For this review, take the finished solid that the model builds, in its own axes (mm). A direction names the side the tool comes from. Round coordinates to 2 decimals unless told otherwise and drop trailing zeros. Order: outer loops, then holes, each group sorted by start corner. A loop starts at its lowest first (then second) coordinate and runs counter-clockwise, first axis right, second up.
```python
from build123d import *

# Parameters (mm, degrees)
EXTRUDE_1_DEPTH     = 1.5
EXTRUDE_2_DEPTH     = 6.5
CUT_EXTRUDE_1_DEPTH = 1
SKETCH_4_R          = 4.015
EXTRUDE_3_DEPTH     = 4
SKETCH_6_R          = 4.015
EXTRUDE_4_DEPTH     = 4
SKETCH_7_R          = 2.4
CUT_EXTRUDE_3_DEPTH = 48.711742668
SKETCH_8_W          = 9
SKETCH_8_H          = 5
EXTRUDE_5_DEPTH     = 8.5
SKETCH_9_W          = 4.5
SKETCH_9_H          = 5
SKETCH_10_R         = 1.75
CUT_EXTRUDE_4_DEPTH = 51.943190951


with BuildPart() as part:
    # 스케치1 → 보스-돌출1 (new body)
    with BuildSketch(Plane(origin=(0, 0, 0), x_dir=(1, 0, 0), z_dir=(0, 1, 0))):
        Polygon((13.776603565, 33.25966317), (-13.776603565, 33.25966317), (-33.25966317, 13.776603565), (-33.25966317, -13.776603565), (-13.776603565, -33.25966317), (13.776603565, -33.25966317), (33.25966317, -13.776603565), (33.25966317, 13.776603565), align=None)
        Polygon((-13.27954729, 32.05966317), (-32.05966317, 13.27954729), (-32.05966317, -13.27954729), (-13.27954729, -32.05966317), (13.27954729, -32.05966317), (32.05966317, -13.27954729), (32.05966317, 13.27954729), (13.27954729, 32.05966317), align=None, mode=Mode.SUBTRACT)
        Polygon((13.27954729, 32.05966317), (-13.27954729, 32.05966317), (-32.05966317, 13.27954729), (-32.05966317, -13.27954729), (-13.27954729, -32.05966317), (13.27954729, -32.05966317), (32.05966317, -13.27954729), (32.05966317, 13.27954729), align=None)
    extrude(amount=EXTRUDE_1_DEPTH)

    # 스케치2 → 보스-돌출2 (add)
    with BuildSketch(Plane.XZ):
        Polygon((-33.25966317, -13.776603565), (-13.776603565, -33.25966317), (13.776603565, -33.25966317), (33.25966317, -13.776603565), (33.25966317, 13.776603565), (13.776603565, 33.25966317), (-13.776603565, 33.25966317), (-33.25966317, 13.776603565), align=None)
        Polygon((-32.05966317, -13.27954729), (-13.27954729, -32.05966317), (13.27954729, -32.05966317), (32.05966317, -13.27954729), (32.05966317, 13.27954729), (13.27954729, 32.05966317), (-13.27954729, 32.05966317), (-32.05966317, 13.27954729), align=None, mode=Mode.SUBTRACT)
        Polygon((-32.05966317, 13.27954729), (-32.05966317, -13.27954729), (-13.27954729, -32.05966317), (13.27954729, -32.05966317), (32.05966317, -13.27954729), (32.05966317, 13.27954729), (13.27954729, 32.05966317), (-13.27954729, 32.05966317), align=None)
        Polygon((-30.85966317, -12.782491015), (-12.782491015, -30.85966317), (12.782491015, -30.85966317), (30.85966317, -12.782491015), (30.85966317, 12.782491015), (12.782491015, 30.85966317), (-12.782491015, 30.85966317), (-30.85966317, 12.782491015), align=None, mode=Mode.SUBTRACT)
        Polygon((-30.85966317, 12.782491015), (-30.85966317, -12.782491015), (-12.782491015, -30.85966317), (12.782491015, -30.85966317), (30.85966317, -12.782491015), (30.85966317, 12.782491015), (12.782491015, 30.85966317), (-12.782491015, 30.85966317), align=None)
        Polygon((-29.65966317, -12.285434741), (-12.285434741, -29.65966317), (12.285434741, -29.65966317), (29.65966317, -12.285434741), (29.65966317, 12.285434741), (12.285434741, 29.65966317), (-12.285434741, 29.65966317), (-29.65966317, 12.285434741), align=None, mode=Mode.SUBTRACT)
    extrude(amount=EXTRUDE_2_DEPTH)

    # 스케치3 → 컷-돌출1 (cut)
    with BuildSketch(Plane.XZ.offset(6.5)):
        Polygon((-32.05966317, -13.27954729), (-13.27954729, -32.05966317), (13.27954729, -32.05966317), (32.05966317, -13.27954729), (32.05966317, 13.27954729), (13.27954729, 32.05966317), (-13.27954729, 32.05966317), (-32.05966317, 13.27954729), align=None)
        Polygon((-30.85966317, -12.782491015), (-12.782491015, -30.85966317), (12.782491015, -30.85966317), (30.85966317, -12.782491015), (30.85966317, 12.782491015), (12.782491015, 30.85966317), (-12.782491015, 30.85966317), (-30.85966317, 12.782491015), align=None, mode=Mode.SUBTRACT)
    extrude(amount=-CUT_EXTRUDE_1_DEPTH, mode=Mode.SUBTRACT)

    # 스케치4 → 보스-돌출3 (add)
    with BuildSketch(Plane(origin=(0, 1.5, 0), x_dir=(1, 0, 0), z_dir=(0, 1, 0))):
        with Locations(Location((0, 0, 0), (0, 0, 270))):
            Circle(SKETCH_4_R)
    extrude(amount=EXTRUDE_3_DEPTH)

    # 스케치6 → 보스-돌출4 (add)
    with BuildSketch(Plane.XZ):
        with Locations(Location((0, 0, 0), (0, 0, 90))):
            Circle(SKETCH_6_R)
    extrude(amount=EXTRUDE_4_DEPTH)

    # 스케치7 → 컷-돌출3 (cut, through all)
    with BuildSketch(Plane(origin=(0, 1.5, 0), x_dir=(1, 0, 0), z_dir=(0, 1, 0))):
        with Locations(Location((0, -27, 0), (0, 0, 270))):
            Circle(SKETCH_7_R)
    extrude(amount=-CUT_EXTRUDE_3_DEPTH, mode=Mode.SUBTRACT)

    # 스케치8 → 보스-돌출5 (add)
    with BuildSketch(Plane(origin=(0, 1.5, 0), x_dir=(1, 0, 0), z_dir=(0, 1, 0))):
        with Locations((-28.75966317, 0)):
            Rectangle(SKETCH_8_W, SKETCH_8_H)
    extrude_5 = extrude(amount=EXTRUDE_5_DEPTH)

    # 스케치9 → 회전1 (revolve)
    with BuildSketch(Plane(origin=(0, 10, 0), x_dir=(1, 0, 0), z_dir=(0, 1, 0))):
        with Locations((-31.00966317, 0)):
            Rectangle(SKETCH_9_W, SKETCH_9_H)
    revolve_1 = revolve(axis=Axis((-28.75966317, 10, -5.508751215), (0, 0, 1)))

    # 스케치10 → 컷-돌출4 (cut, through all)
    with BuildSketch(Plane.XY.offset(2.5)):
        with Locations((-28.75966317, 10)):
            Circle(SKETCH_10_R)
    cut_extrude_4 = extrude(amount=-CUT_EXTRUDE_4_DEPTH, mode=Mode.SUBTRACT)

    # 대칭 복사1: 보스-돌출5, 회전1, 컷-돌출4 across plane
    add(extrude_5.mirror(Plane(origin=(0, 0, 0), x_dir=(0, 0, 1), z_dir=(1, 0, 0))))
    add(revolve_1.mirror(Plane(origin=(0, 0, 0), x_dir=(0, 0, 1), z_dir=(1, 0, 0))))
    add(cut_extrude_4.mirror(Plane(origin=(0, 0, 0), x_dir=(0, 0, 1), z_dir=(1, 0, 0))), mode=Mode.SUBTRACT)


solid = part.part
```
Q1. Take a section at D-D, the plane z = 27. State the section outline as (x, y) points, plus the area to 3 significant figures.
Q2. Take a section at B-B, the plane z = 0. Count the separate pieces of the cut face and the enclosed holes in it, plus the area to 3 significant figures.
Q3. Clearance check with flat-ended pins moving along their axes: pin 1 (4.5 mm diameter, centred on x = 26.5, y = 5, fed in from -Z); pin 2 (1.5 mm diameter, centred on x = -13.5, y = 4, fed in from +Z); pin 3 (12 mm diameter, centred on x = 4.5, y = 10.5, fed in from +Z); pin 4 (6 mm diameter, centred on x = -13, z = 5, fed in from +Y). State where each tip first meets the part, or that it passes through.
Q4. Tool access review of faces 5 (the face through (24.26, 6, 0)), 6 (the face through (29, 8, -2.5)), 7 (the face through (0.106, 0.76, 24.602)), 8 (the face through (29.66, -3, 0)), 9 (the face through (29, 8, 2.5)): name each direction out of +Z, -Z, +X, -X, +Y, -Y from which nothing blocks a thin tool from reaching the whole face with its end or side.
Q5. Take a section at A-A, the plane y = -2.25. State the section outline as (x, z) points (3 decimals), plus the area to 3 significant figures.
Q6. Mouldability with a two-part tool opening along X and no side actions: class faces 1 (the face through (0, 0, -7)), 2 (the face through (0, -2, 33.26)), 3 (the face through (21.69, -6.01, -21.95)), 4 (the face through (33.26, -2, 0)) as +X half, -X half, draft (parallel to the pull), parting line (faces both ways), or undercut.
Q7. Take a section at C-C, the plane x = 0. State the section outline as (y, z) points (3 decimals), plus the area to 3 significant figures.
Q8. Wall thickness on line 1 (Z direction, x = -9.5, y = -1.25); line 2 (Y direction, x = -4, z = -12.5); line 3 (Z direction, x = -30, y = 6.75): over which ranges is each line inside the solid? List them lowest first.
Working result:
1. outline: (-20.04, -6.5) - (-18.34, -6.5) - (-18.34, -5.5) - (-16.64, -5.5) - (-16.64, -6.5) - (-14.95, -6.5) - (-14.95, 0) - (-2.4, 0) - (-2.4, 1.5) - (-20.04, 1.5) - close; (2.4, 0) - (14.95, 0) - (14.95, -6.5) - (16.64, -6.5) - (16.64, -5.5) - (18.34, -5.5) - (18.34, -6.5) - (20.04, -6.5) - (20.04, 1.5) - (2.4, 1.5) - close
1. area: 116 mm2
2. separate pieces: 1
2. enclosed holes: 2
2. area: 406 mm2
3. pin 1: stops at z = -2.5
3. pin 2: passes through
3. pin 3: stops at z = 3.84
3. pin 4: stops at y = 1.5
4. face 5: +Z, -Z, +Y
4. face 6: -Z, +X, +Y
4. face 7: +Y, -Y
4. face 8: -Y
4. face 9: +Z, +X, +Y
5. outline: (-33.26, -13.777) - (-13.777, -33.26) - (13.777, -33.26) - (33.26, -13.777) - (33.26, 13.777) - (13.777, 33.26) - (-13.777, 33.26) - (-33.26, 13.777) - close; circle Ø8.03 at (0, 0); hole (-29.66, -12.285) - (-12.285, -29.66) - (12.285, -29.66) - (29.66, -12.285) - (29.66, 12.285) - (12.285, 29.66) - (-12.285, 29.66) - (-29.66, 12.285) - close
5. area: 801 mm2
6. face 1: undercut
6. face 2: draft
6. face 3: undercut
6. face 4: +X half
7. outline: (-6.5, -33.26) - (1.5, -33.26) - (1.5, -4.015) - (5.5, -4.015) - (5.5, 4.015) - (1.5, 4.015) - (1.5, 24.6) - (0, 24.6) - (0, 4.015) - (-4, 4.015) - (-4, -4.015) - (0, -4.015) - (0, -29.66) - (-6.5, -29.66) - (-6.5, -30.86) - (-5.5, -30.86) - (-5.5, -32.06) - (-6.5, -32.06) - close; (-6.5, 29.66) - (0, 29.66) - (0, 29.4) - (1.5, 29.4) - (1.5, 33.26) - (-6.5, 33.26) - (-6.5, 32.06) - (-5.5, 32.06) - (-5.5, 30.86) - (-6.5, 30.86) - close
7. area: 201 mm2
8. line 1: z = -33.26 to -29.66, 29.66 to 33.26
8. line 2: y = 0 to 1.5
8. line 3: z = -2.5 to 2.5
